```python
from build123d import *

# Parameters (mm, degrees)
BLANKSKE_W        = 302
BLANKSKE_H        = 28
BLANK_DEPTH       = 20
TOOTHCUTSIM_DEPTH = 304.95394388
TEETHCUTS_COUNT   = 25
TEETHCUTS_PITCH   = 12.5663706


with BuildPart() as part:
    # BlankSke → Blank (new body)
    with BuildSketch(Plane.XY):
        with Locations((151, 14)):
            Rectangle(BLANKSKE_W, BLANKSKE_H)
    extrude(amount=-BLANK_DEPTH)

    # TooCutSkeSim → ToothCutSim (cut, through all)
    with BuildSketch(Plane.XY):
        Polygon((1.702741479, 19), (-1.702741479, 19), (-4.987718431, 28.0254), (4.987718431, 28.0254), align=None)
    toothcutsim = extrude(amount=-TOOTHCUTSIM_DEPTH, mode=Mode.SUBTRACT)

    # TeethCuts: ToothCutSim ×25
    with Locations(*[(i * TEETHCUTS_PITCH, 0, 0) for i in range(1, TEETHCUTS_COUNT)]):
        add(toothcutsim, mode=Mode.SUBTRACT)


solid = part.part
```
Geometry: final body of the model. Coordinates: model frame, mm. A direction names the side the tool comes from. Coordinates: 2 decimals unless noted, no trailing zeros.
Item 1: Contact query for flat-ended pins moving along their axis: P1, Ø2.5, axis at x = 88, z = -11.5, coming from the +Y side; P2, Ø4, axis at y = 22, z = -12.5, coming from the -X side. Output: stop coordinate, or through.
Answer:
P1: stops at y = 19
P2: stops at x = 2.07
Item 2: Material intervals for line 1 along Y through (x, z) = (165, -17.25), sorted ascending.
Answer:
line 1: y = 0 to 19
Item 3: Section query A-A (y = 22). State how many separate pieces and enclosed holes the cut face has, then the cut area to 3 significant figures.
Answer:
separate pieces: 24
enclosed holes: 0
area: 3,350 mm2
Item 4: Access query for faces 1 (the face through (72.08, 23.44, -9.86)), 2 (the face through (3.364, 23.563, -9.86)). Directions: +Z, -Z, +X, -X, +Y, -Y. A direction counts if a zero-diameter tool reaches every point of the face in a straight line with its end or side. Return the directions, or none.
Answer:
face 1: +Z, -Z, +Y
face 2: +Z, -Z, -X, +Y
